Work out the finished part from the listing and answer in its coordinate system (mm). Give positions to 0.01 mm unless a question says otherwise; leave off trailing zeros. Write each loop counter-clockwise with the first axis right and the second up, starting at its lowest first coordinate (ties: lowest second). Pieces come first, ordered by that corner, then holes.
1) Determine the mould class of faces 1 (the face through (-0.13, 30.82, 2.54)), 2 (the face through (-18, 26, 5)), 3 (the face through (-7.944, 43.799, 2.465)) for opening direction Y: pulls with the +Y half, pulls with the -Y half, needs draft (parallel to the pull), parting line crosses it, or undercut.
2) Find section B-B (z = 2.3). Determine the outline of the cut face in (x, y).
3) Given pin 1 Ø2 at (y, z) = (20, 2.5) entering from +X; pin 2 Ø3.5 at (x, y) = (-7.5, 45.8) entering from -Z, each flat-ended and moving along its own axis, determine where each tip first touches the part or whether it passes through.
4) Find section D-D (x = -33.5). Determine the outline of the cut face in (y, z), plus the area to 3 significant figures.
5) Straight lines are drawn through the part: probe 1 along Y at (x, z) = (-7.5, 4); probe 2 along X at (y, z) = (36, 4.05); probe 3 along Y at (x, z) = (-8.5, 3.6). For each, find the intervals that lie inside material, in ascending order.
6) Find section A-A (x = -7.5). Determine the outline of the cut face in (y, z), plus the area to 3 significant figures.
7) Find section C-C (y = 35.8). Determine the outline of the cut face in (x, z), plus the area to 4 significant figures.
```python
from build123d import *

# Parameters (mm, degrees)
SKETCH_1_R      = 6
SKETCH_1_R_2    = 2.05
EXTRUDE_1_DEPTH = 5
FILLET_1_R      = 3


with BuildPart() as part:
    # ｽｹｯﾁ1 → ﾎﾞｽ - 押し出し1 (new body)
    with BuildSketch(Plane.XY):
        Polygon((-36, 0), (-20, 0), (0, 30.8), (0, 50.8), (-15, 50.8), (-36, 28.3), align=None)
        with Locations((-28, 14.15)):
            Circle(SKETCH_1_R, mode=Mode.SUBTRACT)
        with Locations((-7.5, 35.8)):
            Circle(SKETCH_1_R_2, mode=Mode.SUBTRACT)
        with Locations((-7.5, 45.8)):
            Circle(SKETCH_1_R_2, mode=Mode.SUBTRACT)
    extrude(amount=EXTRUDE_1_DEPTH)

    # ﾌｨﾚｯﾄ1
    fillet_1_edges = [part.edges().sort_by_distance(p)[0] for p in [
        (-15, 50.8, 2.5),
        (0, 50.8, 2.5),
        (0, 30.8, 2.5),
        (-20, 0, 2.5),
        (-36, 0, 2.5),
        (-36, 28.3, 2.5),
    ]]
    fillet(fillet_1_edges, radius=FILLET_1_R)


solid = part.part
```
Results:
1. face 1: pulls with the -Y half
1. face 2: needs draft
1. face 3: undercut
2. outline: (-36, 3) arc R3 ccw to (-33, 0) - (-21.63, 0) arc R3 ccw to (-19.11, 1.37) - (-0.48, 30.05) arc R3 ccw to (0, 31.69) - (0, 47.8) arc R3 ccw to (-3, 50.8) - (-13.7, 50.8) arc R3 ccw to (-15.89, 49.85) - (-35.19, 29.16) arc R3 ccw to (-36, 27.12) - close; hole circle Ø12 at (-28, 14.15); hole circle Ø4.1 at (-7.5, 35.8); hole circle Ø4.1 at (-7.5, 45.8)
3. pin 1: stops at x = -6.36
3. pin 2: passes through
4. outline: (0.04, 0) - (11.75, 0) - (11.75, 5) - (0.04, 5) - close; (16.55, 0) - (30.98, 0) - (30.98, 5) - (16.55, 5) - close
4. area: 131 mm2
5. probe 1: y = 19.25 to 33.75, 37.85 to 43.75, 47.85 to 50.8
5. probe 2: x = -28.81 to -9.54, -5.46 to 0
5. probe 3: y = 17.71 to 34.01, 37.59 to 44.01, 47.59 to 50.8
6. outline: (19.25, 0) - (33.75, 0) - (33.75, 5) - (19.25, 5) - close; (37.85, 0) - (43.75, 0) - (43.75, 5) - (37.85, 5) - close; (47.85, 0) - (50.8, 0) - (50.8, 5) - (47.85, 5) - close
6. area: 117 mm2
7. outline: (-29, 0) - (-9.55, 0) - (-9.55, 5) - (-29, 5) - close; (-5.45, 0) - (0, 0) - (0, 5) - (-5.45, 5) - close
7. area: 124.5 mm2
